Could you check a few things on this drawing? It's one solid part, dimensions in mm from its lowest x, y, z. Coordinates: 2 decimals unless noted, no trailing zeros. Order: outer loops, then holes, each group sorted by start corner. A loop starts at its lowest first (then second) coordinate and runs counter-clockwise, first axis right, second up. Notation, with made-up numbers: (46.25, 74.5) - (64.25, 74.5) arc R21 cw to (64.25, 81.5) - close; hole circle Ø4 at (64.5, -3). An arc over 180 degrees is marked (long way). Answer in a Markdown table with one row per item. Add a question column.
Item 1: I want a section at C-C (z = 0.7). Please give me the cut outline in (x, y), plus the area to 3 significant figures.
Item 2: Will these pins go through, and if not, where does the flat tip stop? pin 1 Ø1.5 at (y, z) = (19, 1) entering from -X; pin 2 Ø3.5 at (x, y) = (127, 71) entering from +Z.
Item 3: If I drill on line 1 along X through (y, z) = (71, 1.7); line 2 along Y through (x, z) = (127, 1.9); line 3 along X through (y, z) = (12, 0.4), over which ranges is the centre line in solid material (lowest first)? Write a range as from..to.
Item 4: I want a section at A-A (y = 24.5). Please give me the cut outline in (x, z), plus the area to 3 significant figures.
Item 5: I want a section at B-B (x = 69). Please give me the cut outline in (y, z).
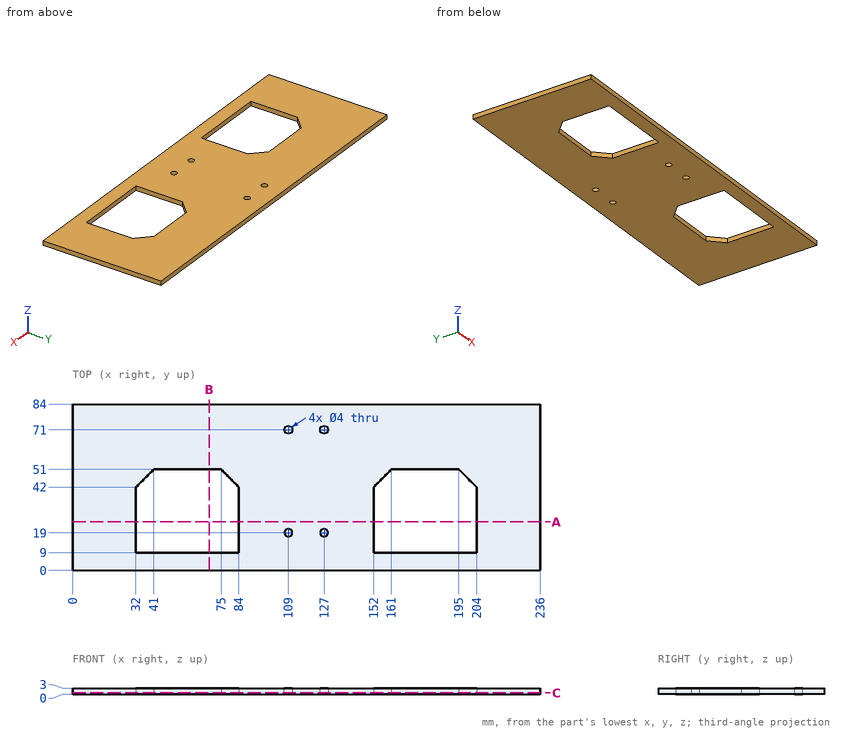
Values follow:
| question | item | result |
|---|---|---|
| 1 | outline | (0, 0) - (236, 0) - (236, 84) - (0, 84) - close; hole (32, 9) - (84, 9) - (84, 42) - (75, 51) - (41, 51) - (32, 42) - close; hole circle Ø4 at (109, 19); hole circle Ø4 at (109, 71); hole circle Ø4 at (127, 19); hole circle Ø4 at (127, 71); hole (152, 9) - (204, 9) - (204, 42) - (195, 51) - (161, 51) - (152, 42) - close |
| 1 | area | 15,600 mm^2 |
| 2 | pin 1 | stops at x = 0 |
| 2 | pin 2 | passes through |
| 3 | line 1 | x = 0..107, 111..125, 129..236 |
| 3 | line 2 | y = 0..17, 21..69, 73..84 |
| 3 | line 3 | x = 0..32, 84..152, 204..236 |
| 4 | outline | (0, 0) - (32, 0) - (32, 3) - (0, 3) - close; (84, 0) - (152, 0) - (152, 3) - (84, 3) - close; (204, 0) - (236, 0) - (236, 3) - (204, 3) - close |
| 4 | area | 396 mm^2 |
| 5 | outline | (0, 0) - (9, 0) - (9, 3) - (0, 3) - close; (51, 0) - (84, 0) - (84, 3) - (51, 3) - close |
